Part model, mm, in its own coordinate system. A direction names the side the tool comes from. Round coordinates to 2 decimals unless told otherwise and drop trailing zeros. Order: outer loops, then holes, each group sorted by start corner. A loop starts at its lowest first (then second) coordinate and runs counter-clockwise, first axis right, second up. Notation, with made-up numbers: (42.25, 51.25) - (63.25, 51.25) arc R17 ccw to (63.25, 63.25) - close; hole circle Ø5 at (-17.5, 52). An arc over 180 degrees is marked (long way). Return JSON: item names as keys, results as strings. Group by question number.
Item 1: Probe probe 1 along X at (y, z) = (-90, 1.75); probe 2 along Y at (x, z) = (-50, 3.6); probe 3 along X at (y, z) = (-76, 4.75). List the from-to ranges inside material, lowest first.
Item 2: Drop flat-ended pins along their axis: pin 1 (14.5 mm diameter, centred on x = -21, y = -80.5, fed in from +Z); pin 2 (11 mm diameter, centred on x = 47.5, y = -71.5, fed in from +Z); pin 3 (2 mm diameter, centred on x = -52, z = 6, fed in from +Y). Give the stop position or say it passes through.
Item 3: Tool access for faces 4 (the face through (-16, -90, 4)), 5 (the face through (-53, -77, 4.9)), 6 (the face through (-46.77, -79.838, 4.444)), 7 (the face through (64, -85, 3)): list every direction of +Z, -Z, +X, -X, +Y, -Y with a clear straight run to the whole face (end or side of a thin tool).
Item 4: Saw through at B-B on y = -72.5. State how many separate pieces and enclosed holes the cut face has, and give its area (3 significant figures).
Item 5: Two-plate mould, pull along Y, no slides. Class faces 1 (the face through (-40, -90, 8.2)), 2 (the face through (6.16, -84.94, 2.03)), 3 (the face through (-54.639, -60.805, 0.135)): released by +Y, released by -Y, zero draft, split by the parting line, or undercut.
Item 6: Saw through at A-A on x = 50. List the corners of the cut face in (y, z), and give its area (3 significant figures).
```python
from build123d import *

# Parameters (mm, degrees)
BOSS_EXTRUDE1_DEPTH = 4
SKETCH6_R           = 7
BOSS_EXTRUDE2_DEPTH = 0.9
SKETCH7_R           = 4.3
CUT_EXTRUDE1_DEPTH  = 20
FILLET1_R           = 20
SKETCH8_W           = 64
SKETCH8_H           = 3
BOSS_EXTRUDE3_DEPTH = 4.2
SKETCH10_W          = 16
SKETCH10_H          = 3
CUT_EXTRUDE2_DEPTH  = 20
SKETCH11_R          = 4.3
SKETCH11_R_2        = 3
SKETCH11_R_3        = 1.75
CUT_EXTRUDE3_DEPTH  = 20
CHAMFER1_SIZE       = 0.5


with BuildPart() as part:
    # Sketch3 → Boss-Extrude1 (new body)
    with BuildSketch(Plane.XY):
        with BuildLine():
            Line((-64, -73.627440537), (-64, -91.627440537))
            Line((-64, -91.627440537), (0, -91.627440537))
            Line((0, -91.627440537), (0, -77.201334505))
            ThreePointArc((0, -77.201334505), (-19.791335437, -74.427796509), (-38.057892518, -66.320863438))
            ThreePointArc((-38.057892518, -66.320863438), (-53.795424565, -60.15173082), (-64, -73.627440537))
        make_face()
    extrude(amount=BOSS_EXTRUDE1_DEPTH)

    # Sketch6 → Boss-Extrude2 (add)
    with BuildSketch(Plane.XY.offset(4)):
        with Locations((-50, -73.627440537)):
            Circle(SKETCH6_R)
    extrude(amount=BOSS_EXTRUDE2_DEPTH)

    # Sketch7 → Cut-Extrude1 (cut)
    with BuildSketch(Plane.XY.offset(4.9)):
        with Locations((-50, -73.627440537)):
            Circle(SKETCH7_R)
    extrude(amount=-CUT_EXTRUDE1_DEPTH, mode=Mode.SUBTRACT)

    # Fillet1
    fillet1_edges = [part.edges().sort_by_distance(p)[0] for p in [
        (-38.057892518, -66.320863438, 2),
    ]]
    fillet(fillet1_edges, radius=FILLET1_R)

    # Sketch8 → Boss-Extrude3 (add)
    with BuildSketch(Plane.XY.offset(4)):
        with Locations((-32, -90.127440537)):
            Rectangle(SKETCH8_W, SKETCH8_H)
    extrude(amount=BOSS_EXTRUDE3_DEPTH)

    # Sketch10 → Cut-Extrude2 (cut)
    with BuildSketch(Plane.XY.offset(8.2)):
        with Locations((-8, -90.127440537)):
            Rectangle(SKETCH10_W, SKETCH10_H)
    extrude(amount=-CUT_EXTRUDE2_DEPTH, mode=Mode.SUBTRACT)

    # Sketch11 → Cut-Extrude3 (cut)
    with BuildSketch(Plane.XY.offset(4)):
        with Locations((-31, -79.186135246)):
            Circle(SKETCH11_R)
        with Locations((-17.14802046, -82.330394565)):
            Circle(SKETCH11_R_2)
        with Locations((-5.779829741, -83.233322768)):
            Circle(SKETCH11_R_3)
    extrude(amount=-CUT_EXTRUDE3_DEPTH, mode=Mode.SUBTRACT)

    # Mirror1: part across plane


with BuildPart() as part_1:
    add(part.part)
    add(part.part.mirror(Plane(origin=(0, -91.627440537, 4), x_dir=(0, 0, 1), z_dir=(-1, 0, 0))))

    # Chamfer1
    chamfer1_edges = [part_1.edges().sort_by_distance(p)[0] for p in [
        (-54.98433008, -60.544762919, 0),
        (0, -77.201334505, 0),
        (-37.007349735, -66.705508667, 0),
        (0, -88.627440537, 0),
        (-16, -90.127440537, 0),
        (-40, -91.627440537, 0),
        (-64, -82.627440537, 0),
        (54.98433008, -60.544762919, 0),
        (64, -82.627440537, 0),
        (40, -91.627440537, 0),
        (37.007349735, -66.705508667, 0),
        (16, -90.127440537, 0),
    ]]
    chamfer(chamfer1_edges, length=CHAMFER1_SIZE)


solid = part_1.part
```
Filled in:
{
 "1": {"probe 1": "x = -64 to -16, 16 to 64", "probe 2": "y = -91.63 to -77.93, -69.33 to -59.63", "probe 3": "x = -56.59 to -53.59, -46.41 to -43.41, 43.41 to 46.41, 53.59 to 56.59"},
 "2": {"pin 1": "stops at z = 4", "pin 2": "stops at z = 4.9", "pin 3": "stops at y = -88.63"},
 "3": {"face 4": "+Z, -Z, -Y", "face 5": "+Z, +X, -X, +Y", "face 6": "+Z", "face 7": "+Z, -Z, +X, +Y, -Y"},
 "4": {"separate pieces": "4", "enclosed holes": "0", "area": "250 mm^2"},
 "5": {"face 1": "zero draft", "face 2": "undercut", "face 3": "released by +Y"},
 "6": {"outline": "(-91.63, 0.5) - (-91.13, 0) - (-77.93, 0) - (-77.93, 4.9) - (-80.63, 4.9) - (-80.63, 4) - (-88.63, 4) - (-88.63, 8.2) - (-91.63, 8.2) - close; (-69.33, 0) - (-60.13, 0) - (-59.63, 0.5) - (-59.63, 4) - (-66.63, 4) - (-66.63, 4.9) - (-69.33, 4.9) - close", "area": "111 mm^2"}
}
